Work out the finished part from the listing and answer in its coordinate system (mm). A direction names the side the tool comes from. Give positions to 0.01 mm unless a question says otherwise; leave off trailing zeros. Loops run counter-clockwise (first coordinate to the right, second up) from the corner with the lowest first, then second, coordinate; pieces in that order, holes last. Notation, with made-up numbers: (43.25, -37) - (60.25, -37) arc R33 cw to (60.25, -7) - close; hole circle Ø10 at (-34, 70.25). An arc over 180 degrees is marked (long way). One line per item, written item: value.
from build123d import *

# Parameters (mm, degrees)
SKETCH2_R           = 1.5
BOSS_EXTRUDE1_DEPTH = 3.18
FILLET1_R           = 1


with BuildPart() as part:
    # Sketch2 → Boss-Extrude1 (new body)
    # profile 1 of 7: a face of its own
    with BuildSketch(Plane.XY):
        with BuildLine():
            Line((20.05, 5), (0, 5))
            ThreePointArc((0, 5), (-5, 0), (0, -5))
            Line((0, -5), (22, -5))
            Line((22, -5), (26.846033211, 1.231244133))
            ThreePointArc((26.846033211, 1.231244133), (25.069509679, 3.946911493), (22, 5))
            Line((22, 5), (20.05, 5))
        make_face()
        with Locations(Location((0, 0, 0), (0, 0, 180))):
            Circle(SKETCH2_R, mode=Mode.SUBTRACT)
        with Locations(Location((22, 0, 0), (0, 0, 180))):
            Circle(SKETCH2_R, mode=Mode.SUBTRACT)
    # profile 2 of 7: a face of its own
    with BuildSketch(Plane.XY):
        with BuildLine():
            Line((46.409029503, 15.837507263), (20.05, 5))
            Line((20.05, 5), (22, 5))
            ThreePointArc((22, 5), (25.069509679, 3.946911493), (26.846033211, 1.231244133))
            Line((26.846033211, 1.231244133), (40.112794076, 6.40528087))
            Line((40.112794076, 6.40528087), (45.93826156, 3.969125944))
            Line((45.93826156, 3.969125944), (47.80157067, 4.695816497))
            Line((47.80157067, 4.695816497), (49.66487978, 5.42250705))
            Line((49.66487978, 5.42250705), (51.528188891, 6.149197603))
            Line((51.528188891, 6.149197603), (53.391498001, 6.875888156))
            Line((53.391498001, 6.875888156), (55.48772075, 7.693415028))
            Line((55.48772075, 7.693415028), (53.852667005, 11.885860526))
            Line((53.852667005, 11.885860526), (46.409029503, 15.837507263))
        make_face()
    # profile 3 of 7: a face of its own
    with BuildSketch(Plane.XY):
        Polygon((47.80157067, 4.695816497), (45.93826156, 3.969125944), (47.097006913, 3.750187123), align=None)
    # profile 4 of 7: a face of its own
    with BuildSketch(Plane.XY):
        Polygon((49.66487978, 5.42250705), (47.80157067, 4.695816497), (48.960316023, 4.476877676), align=None)
    # profile 5 of 7: a face of its own
    with BuildSketch(Plane.XY):
        Polygon((50.823625133, 5.203568229), (51.528188891, 6.149197603), (49.66487978, 5.42250705), align=None)
    # profile 6 of 7: a face of its own
    with BuildSketch(Plane.XY):
        Polygon((52.686934243, 5.930258782), (53.391498001, 6.875888156), (51.528188891, 6.149197603), align=None)
    # profile 7 of 7: a face of its own
    with BuildSketch(Plane.XY):
        Polygon((54.550243354, 6.656949335), (55.48772075, 7.693415028), (53.391498001, 6.875888156), align=None)
    extrude(amount=BOSS_EXTRUDE1_DEPTH)

    # Fillet1
    fillet1_edges = [part.edges().sort_by_distance(p)[0] for p in [
        (22, -5, 1.59),
        (20.05, 5, 1.59),
        (46.409029503, 15.837507263, 1.59),
        (53.852667005, 11.885860526, 1.59),
        (40.112794076, 6.40528087, 1.59),
        (26.846033211, 1.231244133, 1.59),
    ]]
    fillet(fillet1_edges, radius=FILLET1_R)


solid = part.part
1. Section B-B (y = 0) is taken. Write down the section's boundary in (x, z), and give its area (3 significant figures).
Output:
outline: (-5, 0) - (-1.5, 0) - (-1.5, 3.18) - (-5, 3.18) - close; (1.5, 0) - (20.5, 0) - (20.5, 3.18) - (1.5, 3.18) - close; (23.5, 0) - (25.89, 0) - (25.89, 3.18) - (23.5, 3.18) - close
area: 79.1 mm²
2. Section D-D (y = 11) is taken. Write down the section's boundary in (x, z).
Output:
outline: (34.64, 0) - (54.2, 0) - (54.2, 3.18) - (34.64, 3.18) - close
3. Section A-A (z = 1.25) is taken. Write down the section's boundary in (x, y).
Output:
outline: (0, -5) - (21.51, -5) arc R1 ccw to (22.3, -4.61) - (26.68, 1.01) arc R1 cw to (27.1, 1.33) - (39.74, 6.26) arc R1 cw to (40.49, 6.25) - (45.94, 3.97) - (47.1, 3.75) - (47.8, 4.7) - (48.96, 4.48) - (49.66, 5.42) - (50.82, 5.2) - (51.53, 6.15) - (52.69, 5.93) - (53.39, 6.88) - (54.55, 6.66) - (55.49, 7.69) - (53.99, 11.54) arc R1 ccw to (53.52, 12.06) - (46.82, 15.62) arc R1 ccw to (45.97, 15.66) - (20.23, 5.08) arc R1 cw to (19.85, 5) - (0, 5) arc R5 ccw to start; hole circle Ø3 at (0, 0); hole circle Ø3 at (22, 0)
4. The mould has two halves that part along Y. Classify faces 4 (the flat face through (33.28, 10.44, 1.57)), 5 (the cylindrical face through (-1.43, -0.45, 1.57)), 6 (the flat face through (25, 3, 3.18)), 7 (the flat face through (11, -5, 2)): released by +Y, released by -Y, zero draft, split by the parting line, or undercut.
Output:
face 4: released by +Y
face 5: undercut
face 6: zero draft
face 7: released by -Y
5. Find the intervals of material crossed by line 1 along Y through (x, z) = (0, 1.35); line 2 along X through (y, z) = (-1.25, 1.75); line 3 along X through (y, z) = (-0.5, 0.3), in increasing order.
Output:
line 1: y = -5 to -1.5, 1.5 to 5
line 2: x = -4.84 to -0.83, 0.83 to 21.17, 22.83 to 24.92
line 3: x = -4.97 to -1.41, 1.41 to 20.59, 23.41 to 25.5
6. Section C-C (x = 11.5) is taken. Write down the section's boundary in (y, z).
Output:
outline: (-5, 0) - (5, 0) - (5, 3.18) - (-5, 3.18) - close
7. For faces 1 (the flat face through (55.012, 7.168, 1.568)), 2 (the flat face through (10, 5, 2)), 3 (the flat face through (50.236, 5.315, 1.568)), determine the directions among +Z, -Z, +X, -X, +Y, -Y from which every point of the face is accessible in a straight line to the end or side of a thin tool.
Output:
face 1: +Z, -Z, +X, -Y
face 2: +Z, -Z, -X, +Y
face 3: +Z, -Z, -Y
8. A flat-ended cylindrical pin translates along its axis: pin 1 Ø1 at (x, z) = (34, 3) entering from +Y. Find the tip coordinate at first contact, or state that the pin passes through.
Output:
pin 1: stops at y = 10.94
